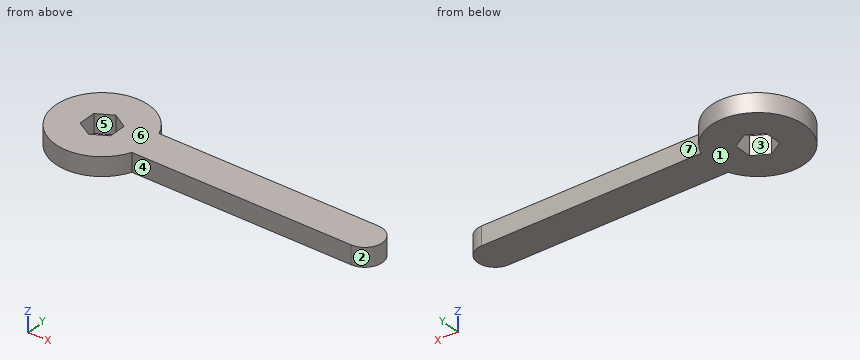
```python
from build123d import *

# Parameters (mm, degrees)
SKETCH_1_R          = 20
EXTRUDE_1_DEPTH     = 8
EXTRUDE_3_DEPTH     = 8
CUT_EXTRUDE_2_DEPTH = 122.918005233


with BuildPart() as part:
    # 草图1 → 凸台-拉伸1 (new body)
    with BuildSketch(Plane.XY):
        Circle(SKETCH_1_R)
    extrude(amount=EXTRUDE_1_DEPTH)

    # 草图4 → 凸台-拉伸3 (add)
    with BuildSketch(Plane.XY):
        with BuildLine():
            Line((0, -7.5), (112.5, -7.5))
            ThreePointArc((112.5, -7.5), (120, 0), (112.5, 7.5))
            Line((112.5, 7.5), (0, 7.5))
            ThreePointArc((0, 7.5), (-7.5, 0), (0, -7.5))
        make_face()
    extrude(amount=EXTRUDE_3_DEPTH)

    # 草图5 → 切除-拉伸2 (cut, through all)
    with BuildSketch(Plane.XY):
        Polygon((6.5, 3.75277675), (0, 7.505553499), (-6.5, 3.75277675), (-6.5, -3.75277675), (0, -7.505553499), (6.5, -3.75277675), align=None)
    extrude(amount=CUT_EXTRUDE_2_DEPTH, mode=Mode.SUBTRACT)


solid = part.part
```
Geometry: final body of the model. Coordinates: model frame, mm. Face numbers are marked on the shaded views. A direction names the side the tool comes from. Give positions to 0.01 mm unless a question says otherwise; leave off trailing zeros. Write each loop counter-clockwise with the first axis right and the second up, starting at its lowest first coordinate (ties: lowest second). Pieces come first, ordered by that corner, then holes.
1. Pin query (flat end, axial travel): P1, Ø1.5, axis at x = 30, z = 6, coming from the +Y side. Return the tip coordinate at first contact, or that it passes through.
2. Section query A-A, the plane y = 0. Return loops of the section in (x, z).
3. Reachability of the marked faces 5, 6 and 7 from +Z, -Z, +X, -X, +Y, -Y: full face, straight path, thin tool, end or side. Return the list, or none.
4. Section query D-D, the plane y = 16. Return loops of the section in (x, z), then the cut area to 3 significant figures.
5. Line query: probe 1 along Y at (x, z) = (67, 3.5); probe 2 along X at (y, z) = (3, 4); probe 3 along Y at (x, z) = (-2, 2). Output: solid intervals per line, ascending.
6. Section query B-B, the plane z = 5. Return loops of the section in (x, y).
7. Section query C-C, the plane x = 55.5. Return loops of the section in (y, z), then the cut area to 3 significant figures.
8. Draft query along Y for the marked faces 1, 2, 3 and 4. Return one class per face: released by +Y, released by -Y, zero draft, split by the parting line, or undercut.
Computed:
1. P1: stops at y = 7.5
2. outline: (-20, 0) - (-6.5, 0) - (-6.5, 8) - (-20, 8) - close; (6.5, 0) - (120, 0) - (120, 8) - (6.5, 8) - close
3. face 5: +Z, -Z
3. face 6: +Z, +X, -X, +Y, -Y
3. face 7: +Z, -Z, +X, +Y
4. outline: (-12, 0) - (12, 0) - (12, 8) - (-12, 8) - close
4. area: 192 mm2
5. probe 1: y = -7.5 to 7.5
5. probe 2: x = -19.77 to -6.5, 6.5 to 119.37
5. probe 3: y = -19.9 to -6.35, 6.35 to 19.9
6. outline: (18.54, -7.5) - (112.5, -7.5) arc R7.5 ccw to (112.5, 7.5) - (18.54, 7.5) arc R20 ccw (long way) to start; hole (-6.5, -3.75) - (0, -7.51) - (6.5, -3.75) - (6.5, 3.75) - (0, 7.51) - (-6.5, 3.75) - close
7. outline: (-7.5, 0) - (7.5, 0) - (7.5, 8) - (-7.5, 8) - close
7. area: 120 mm2
8. face 1: zero draft
8. face 2: split by the parting line
8. face 3: undercut
8. face 4: released by -Y
